```python
from build123d import *

# Parameters (mm, degrees)
CROQUIS1_R              = 27.65
SALIENTE_EXTRUIR1_DEPTH = 5
CROQUIS2_R              = 2.25
SALIENTE_EXTRUIR2_DEPTH = 9.8
CROQUIS8_R              = 19.936300619
CORTAR_EXTRUIR8_DEPTH   = 52.356476321
CHAFL_N1_SIZE           = 1
CROQUIS14_R             = 2.9
CORTAR_EXTRUIR15_DEPTH  = 3
CROQUIS15_R             = 5.5
CORTAR_EXTRUIR16_DEPTH  = 3
CROQUIS16_R             = 1.5
CORTAR_EXTRUIR17_DEPTH  = 25
CROQUIS18_R             = 2.9
CORTAR_EXTRUIR18_DEPTH  = 3
CROQUIS19_R             = 5.5
CORTAR_EXTRUIR19_DEPTH  = 3
CROQUIS20_R             = 1.5
CORTAR_EXTRUIR20_DEPTH  = 22
CORTAR_EXTRUIR21_START  = -2
CORTAR_EXTRUIR21_DEPTH  = 2


with BuildPart() as part:
    # Croquis1 → Saliente-Extruir1 (new body)
    with BuildSketch(Plane.XY):
        Circle(CROQUIS1_R)
    extrude(amount=SALIENTE_EXTRUIR1_DEPTH)

    # Croquis2 → Saliente-Extruir2 (add)
    # profile 1 of 2: a face of its own
    with BuildSketch(Plane(origin=(0, 0, 0), x_dir=(-1, 0, 0), z_dir=(0, 0, -1))):
        with BuildLine():
            ThreePointArc((-32.903550176, 15.136150236), (-36.88979451, 10.508157001), (-33.425205403, 5.477740757))
            Line((-33.425205403, 5.477740757), (-27.421093943, 3.550507988))
            ThreePointArc((-27.421093943, 3.550507988), (-22.324820018, 16.313335379), (-11.713593891, 25.046241598))
            Line((-11.713593891, 25.046241598), (-32.903550176, 15.136150236))
        make_face()
        with Locations((-31.89707142, 10.238497685)):
            Circle(CROQUIS2_R, mode=Mode.SUBTRACT)
    # profile 2 of 2: a face of its own
    with BuildSketch(Plane(origin=(0, 0, 0), x_dir=(-1, 0, 0), z_dir=(0, 0, -1))):
        with BuildLine():
            ThreePointArc((27.65, 0), (23.501050206, -14.567880396), (12.299320852, -24.763868974))
            Line((12.299320852, -24.763868974), (28.440475678, -29.944945762))
            Line((28.440475678, -29.944945762), (30.192362506, -24.487108002))
            Line((30.192362506, -24.487108002), (33.190053815, -15.148084182))
            ThreePointArc((33.190053815, -15.148084182), (36.731135944, -11.790162344), (35.805913272, -6.998621389))
            Line((35.805913272, -6.998621389), (38.863217361, 2.52612041))
            Line((38.863217361, 2.52612041), (40.555491409, 7.798240191))
            Line((40.555491409, 7.798240191), (24.414336583, 12.979316979))
            ThreePointArc((24.414336583, 12.979316979), (26.828892136, 6.688276814), (27.65, 0))
        make_face()
        with Locations((31.89707142, -10.238497685)):
            Circle(CROQUIS2_R, mode=Mode.SUBTRACT)
    extrude(amount=-SALIENTE_EXTRUIR2_DEPTH)

    # Croquis8 → Cortar-Extruir8 (cut, through all)
    with BuildSketch(Plane(origin=(0, 0, 0), x_dir=(-1, 0, 0), z_dir=(0, 0, -1))):
        Circle(CROQUIS8_R)
    extrude(amount=-CORTAR_EXTRUIR8_DEPTH, mode=Mode.SUBTRACT)

    # Chaflán1
    chafl_n1_edges = [part.edges().sort_by_distance(p)[0] for p in [
        (-29.64707142, -10.238497685, 0),
        (34.14707142, 10.238497685, 0),
    ]]
    chamfer(chafl_n1_edges, length=CHAFL_N1_SIZE)

    # Croquis14 → Cortar-Extruir15 (cut)
    with BuildSketch(Plane(origin=(-34.497983543, -11.073352785, 0), x_dir=(0, 0, -1), z_dir=(0.9521513856630914, 0.30562679656707925, 0))):
        with Locations((-7.77864737, 12.203434568)):
            Circle(CROQUIS14_R)
    extrude(amount=CORTAR_EXTRUIR15_DEPTH, mode=Mode.SUBTRACT)

    # Croquis15 → Cortar-Extruir16 (cut)
    with BuildSketch(Plane(origin=(-32.022389941, -10.278723114, 0), x_dir=(0, 0, 1), z_dir=(-0.9521513856630914, -0.30562679656707925, 0))):
        with Locations((7.77864737, 12.203434568)):
            Circle(CROQUIS15_R)
    extrude(amount=-CORTAR_EXTRUIR16_DEPTH, mode=Mode.SUBTRACT)

    # Croquis16 → Cortar-Extruir17 (cut)
    with BuildSketch(Plane(origin=(-29.546796338, -9.484093443, 0), x_dir=(0, 0, -1), z_dir=(0.9521513856630914, 0.30562679656707925, 0))):
        with Locations(Location((-7.77864737, 12.203434568, 0), (0, 0, 270))):
            Circle(CROQUIS16_R)
    extrude(amount=CORTAR_EXTRUIR17_DEPTH, mode=Mode.SUBTRACT)

    # Croquis18 → Cortar-Extruir18 (cut)
    with BuildSketch(Plane(origin=(-34.497983543, -11.073352785, 0), x_dir=(0, 0, -1), z_dir=(0.9521513856630915, 0.30562679656707936, 0))):
        with Locations((-7.867235226, -11.925798003)):
            Circle(CROQUIS18_R)
    extrude(amount=CORTAR_EXTRUIR18_DEPTH, mode=Mode.SUBTRACT)

    # Croquis19 → Cortar-Extruir19 (cut)
    with BuildSketch(Plane(origin=(-32.022389941, -10.278723114, 0), x_dir=(0, 0, 1), z_dir=(-0.9521513856630915, -0.30562679656707936, 0))):
        with Locations((7.867235226, -11.925798003)):
            Circle(CROQUIS19_R)
    extrude(amount=-CORTAR_EXTRUIR19_DEPTH, mode=Mode.SUBTRACT)

    # Croquis20 → Cortar-Extruir20 (cut)
    with BuildSketch(Plane(origin=(-29.546796338, -9.484093443, 0), x_dir=(0, 0, -1), z_dir=(0.9521513856630915, 0.30562679656707936, 0))):
        with Locations(Location((-7.867235226, -11.925798003, 0), (0, 0, 270))):
            Circle(CROQUIS20_R)
    extrude(amount=CORTAR_EXTRUIR20_DEPTH, mode=Mode.SUBTRACT)

    # Croquis21 → Cortar-Extruir21 (cut)
    with BuildSketch(Plane.XY.offset(9.8).offset(CORTAR_EXTRUIR21_START)):
        with BuildLine():
            Line((-25.979532538, -19.288780739), (-25.062652149, -22.145234896))
            Line((-25.062652149, -22.145234896), (-18.911821549, -20.170907409))
            ThreePointArc((-18.911821549, -20.170907409), (-20.090955919, -18.996736306), (-21.19732255, -17.753760635))
            Line((-21.19732255, -17.753760635), (-25.979532538, -19.288780739))
        make_face()
        with BuildLine():
            Line((-33.354072593, 3.685901488), (-32.437192203, 0.829447331))
            Line((-32.437192203, 0.829447331), (-27.545683066, 2.399550877))
            ThreePointArc((-27.545683066, 2.399550877), (-27.350119986, 4.061211244), (-27.05441226, 5.708001162))
            Line((-27.05441226, 5.708001162), (-33.354072593, 3.685901488))
        make_face()
        Polygon((-39.113997867, 3.307403367), (-37.341362447, -2.21507467), (-34.865768845, -1.420444999), (-36.638404265, 4.102033038), align=None)
        Polygon((-31.739457813, -19.66727886), (-29.966822393, -25.189756897), (-27.491228791, -24.395127226), (-29.263864211, -18.872649189), align=None)
    extrude(amount=CORTAR_EXTRUIR21_DEPTH, mode=Mode.SUBTRACT)


solid = part.part
```
Input: part model. Units: mm. Frame: model coordinates. A direction names the side the tool comes from. Round coordinates to 2 decimals unless told otherwise and drop trailing zeros. Loops run counter-clockwise (first coordinate to the right, second up) from the corner with the lowest first, then second, coordinate; pieces in that order, holes last. Notation, with made-up numbers: (-9.75, 18.5) - (35.25, 18.5) arc R32 cw to (35.25, 51.5) - close; hole circle Ø4 at (71.5, 24). An arc over 180 degrees is marked (long way). One line per item, written item: value. Start each with the question number.
(1) Section B-B, the plane y = 17. Return loops of the section in (x, z), plus the area to 3 significant figures.
(2) Access query for faces 1 (the flat face through (-36.121, -1.823, 8.786)), 2 (the cylindrical face through (-10.72, 16.81, 2.46)), 3 (the flat face through (-30.2, 4.7, 8.8)). Directions: +Z, -Z, +X, -X, +Y, -Y. A direction counts if a zero-diameter tool reaches every point of the face in a straight line with its end or side. Return the directions, or none.
(3) Section A-A, the plane x = 0. Return loops of the section in (y, z).
(4) Contact query for flat-ended pins moving along their axis: P1, Ø5, axis at y = 18, z = 1.5, coming from the +X side; P2, Ø3, axis at y = -18, z = 8.5, coming from the -X side; P3, Ø6, axis at x = -31.9, y = -10.24, coming from the -Z side. Output: stop coordinate, or through.
(5) Draft query along Y for faces 4 (the cylindrical face through (-8.48, 26.317, 2.465)), 5 (the flat face through (-28.75, -24.8, 8.79)), 6 (the cylindrical face through (29.75, 10.91, 5.34)), 7 (the flat face through (-32, 8, 9.8)). Return one class per face: +Y half, -Y half, draft (parallel to the pull), parting line (faces both ways), or undercut.
(6) Ray query, line 1 (Y direction, x = 0, z = 3.75); line 2 (X direction, y = -9, z = 2.5); line 3 (X direction, y = 18.5, z = 3). Return the intervals inside material, ascending. Write a range as [from, to].
(7) Section C-C, the plane x = -15.5. Return loops of the section in (y, z).
Results below:
1. outline: (-21.81, 0) - (-10.41, 0) - (-10.41, 5) - (-21.81, 5) - close; (10.41, 0) - (28.92, 0) - (28.92, 9.8) - (21.81, 9.8) - (21.81, 5) - (10.41, 5) - close
1. area: 184 mm^2
2. face 1: +Z, -X
2. face 2: +Z, -Z
2. face 3: +Z
3. outline: (-27.65, 0) - (-19.94, 0) - (-19.94, 5) - (-27.65, 5) - close; (19.94, 0) - (27.65, 0) - (27.65, 5) - (19.94, 5) - close
4. P1: x = 32.13
4. P2: x = -32.76
4. P3: z = 0.25
5. face 4: +Y half
5. face 5: undercut
5. face 6: undercut
5. face 7: draft
6. line 1: [-27.65, -19.94], [19.94, 27.65]
6. line 2: [-36.82, -33.78], [-30.02, -17.79], [17.79, 26.14]
6. line 3: [-20.55, -7.43], [7.43, 25.71]
7. outline: (-25.79, 0) - (-12.54, 0) - (-12.54, 5) - (-22.9, 5) - (-22.9, 9.8) - (-25.79, 9.8) - close; (12.54, 0) - (22.9, 0) - (22.9, 5) - (12.54, 5) - close
